Verification items for the finished model (mm, model axes). Face numbers are marked on the shaded views. A direction names the side the tool comes from. Give positions to 0.01 mm unless a question says otherwise; leave off trailing zeros. Order: outer loops, then holes, each group sorted by start corner. A loop starts at its lowest first (then second) coordinate and runs counter-clockwise, first axis right, second up. Notation, with made-up numbers: (42, 3.25) -> (49, 3.25) arc R30 cw to (49, 28.25) -> close; hole circle Ø3 at (4.5, -37.75). An arc over 180 degrees is marked (long way). Return JSON: item names as keys, results as strings. Group by question number.
(1) Tool access check on the marked faces 1 and 2. Record the directions out of +Z, -Z, +X, -X, +Y, -Y that give a thin tool (end or side, any length) a straight path to the whole face; none if there is none.
(2) Cross-section at C-C on x = -1.75. Enter the section's corners in (y, z).
(3) Cross-section at A-A on y = 0. Enter the section's corners in (x, z).
(4) Release check for a two-part mould opening along Y. For the marked faces 3, 4 and 5 record: pulls with the +Y half, pulls with the -Y half, needs draft (parallel to the pull), parting line crosses it, or undercut.
(5) Cross-section at D-D on y = 2.25. Enter the section's corners in (x, z), then the cut area to 3 significant figures.
(6) Depth check by flat-ended pin: pin 1 Ø3.5 at (x, y) = (0, 0) entering from +Z. Enter the tip coordinate at first touch or a pass-through.
(7) Thickness scan on line 1 along Y through (x, z) = (0, 1.3); line 2 along Z through (x, y) = (-2.5, -1); line 3 along X through (y, z) = (-0.75, 0.15). Record the ranges inside material, lowest first.
from build123d import *

# Parameters (mm, degrees)
SKETCH1_R               = 3.75
BOSS_EXTRUDE2_DEPTH     = 1.5
SKETCH2_R               = 2.5
BOSS_EXTRUDE3_DEPTH     = 0.5
SKETCH3_R               = 1.5
CUT_EXTRUDE2_DEPTH      = 1
CUT_EXTRUDE2_DEPTH_BACK = 3


with BuildPart() as part:
    # Sketch1 → Boss-Extrude2 (new body)
    with BuildSketch(Plane.XY):
        Circle(SKETCH1_R)
    extrude(amount=BOSS_EXTRUDE2_DEPTH)

    # Sketch2 → Boss-Extrude3 (add)
    with BuildSketch(Plane.XY.offset(1.5)):
        Circle(SKETCH2_R)
    extrude(amount=BOSS_EXTRUDE3_DEPTH)

    # Sketch3 → Cut-Extrude2 (cut, two sides)
    with BuildSketch(Plane.XY.offset(2)) as cut_extrude2_sk:
        Circle(SKETCH3_R)
    extrude(amount=CUT_EXTRUDE2_DEPTH, mode=Mode.SUBTRACT)
    extrude(cut_extrude2_sk.sketch, amount=-CUT_EXTRUDE2_DEPTH_BACK, mode=Mode.SUBTRACT)


solid = part.part
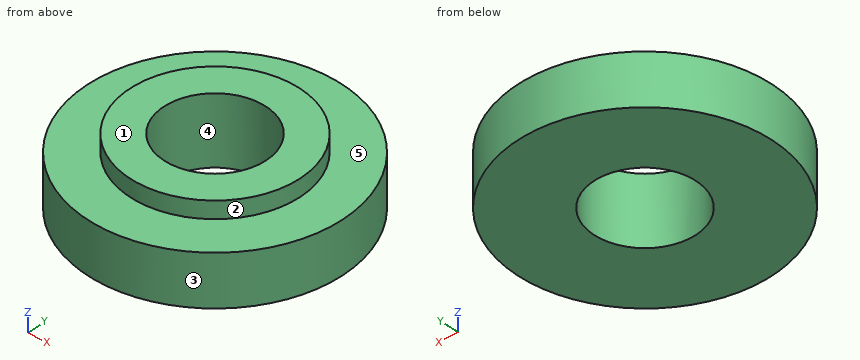
Verdict:
{
 "1": {"face 1": "+Z, +X, -X, +Y, -Y", "face 2": "+Z"},
 "2": {"outline": "(-3.32, 0) -> (3.32, 0) -> (3.32, 1.5) -> (1.79, 1.5) -> (1.79, 2) -> (-1.79, 2) -> (-1.79, 1.5) -> (-3.32, 1.5) -> close"},
 "3": {"outline": "(-3.75, 0) -> (-1.5, 0) -> (-1.5, 2) -> (-2.5, 2) -> (-2.5, 1.5) -> (-3.75, 1.5) -> close; (1.5, 0) -> (3.75, 0) -> (3.75, 1.5) -> (2.5, 1.5) -> (2.5, 2) -> (1.5, 2) -> close"},
 "4": {"face 3": "parting line crosses it", "face 4": "undercut", "face 5": "needs draft"},
 "5": {"outline": "(-3, 0) -> (3, 0) -> (3, 1.5) -> (1.09, 1.5) -> (1.09, 2) -> (-1.09, 2) -> (-1.09, 1.5) -> (-3, 1.5) -> close", "area": "10.1 mm²"},
 "6": {"pin 1": "z = 2"},
 "7": {"line 1": "-3.75 to -1.5, 1.5 to 3.75", "line 2": "0 to 1.5", "line 3": "-3.67 to -1.3, 1.3 to 3.67"}
}
